Check sheet for the drawn part. Datum: minimum x, y, z corner. Units: mm. Coordinates: 2 decimals unless noted, no trailing zeros. Write each loop counter-clockwise with the first axis right and the second up, starting at its lowest first coordinate (ties: lowest second). Pieces come first, ordered by that corner, then holes. Notation, with made-up numbers: (4.5, -36.75) -> (61.5, -36.75) arc R17 cw to (61.5, -18.75) -> close; hole circle Ø4 at (55, -1). An arc over 180 degrees is marked (long way). Write each question's results on one line, items separated by ' | '. Start each with the question number.
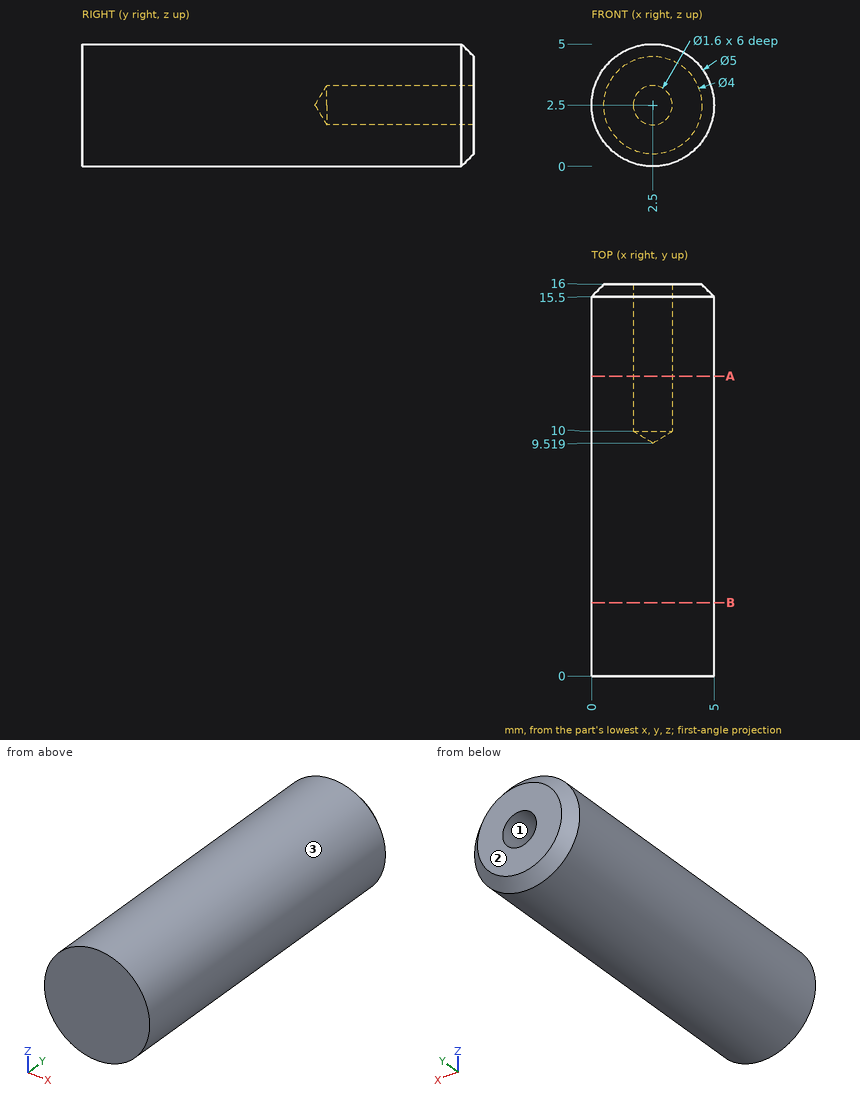
1. Sectioned sample at A-A on y = 12.25. Record the cut outline in (x, z), plus the area to 3 significant figures.
2. Mould release check, pull along Z, two halves, no side actions. Record for the marked faces 1, 2 and 3: +Z half, -Z half, draft (parallel to the pull), parting line (faces both ways), or undercut.
3. Material ranges on probe 1 along Z at (x, y) = (2.5, 14.25); probe 2 along Z at (x, y) = (4.4, 12) (1 decimal), recorded low to high. Write a range as from..to.
4. Depth check by flat-ended pin: pin 1 Ø1.5 at (y, z) = (14, 3.5) entering from +X; pin 2 Ø2 at (y, z) = (2.5, 0.5) entering from -X. Enter the tip coordinate at first touch or a pass-through.
5. Sectioned sample at B-B on y = 3. Record the cut outline in (x, z).
Computed values:
1) outline: circle Ø5 at (2.5, 2.5); hole circle Ø1.6 at (2.5, 2.5) | area: 17.6 mm^2
2) face 1: undercut | face 2: draft | face 3: parting line
3) probe 1: z = 0..1.7, 3.3..5 | probe 2: z = 0.9..4.1
4) pin 1: stops at x = 4.99 | pin 2: stops at x = 0.21
5) outline: circle Ø5 at (2.5, 2.5)
